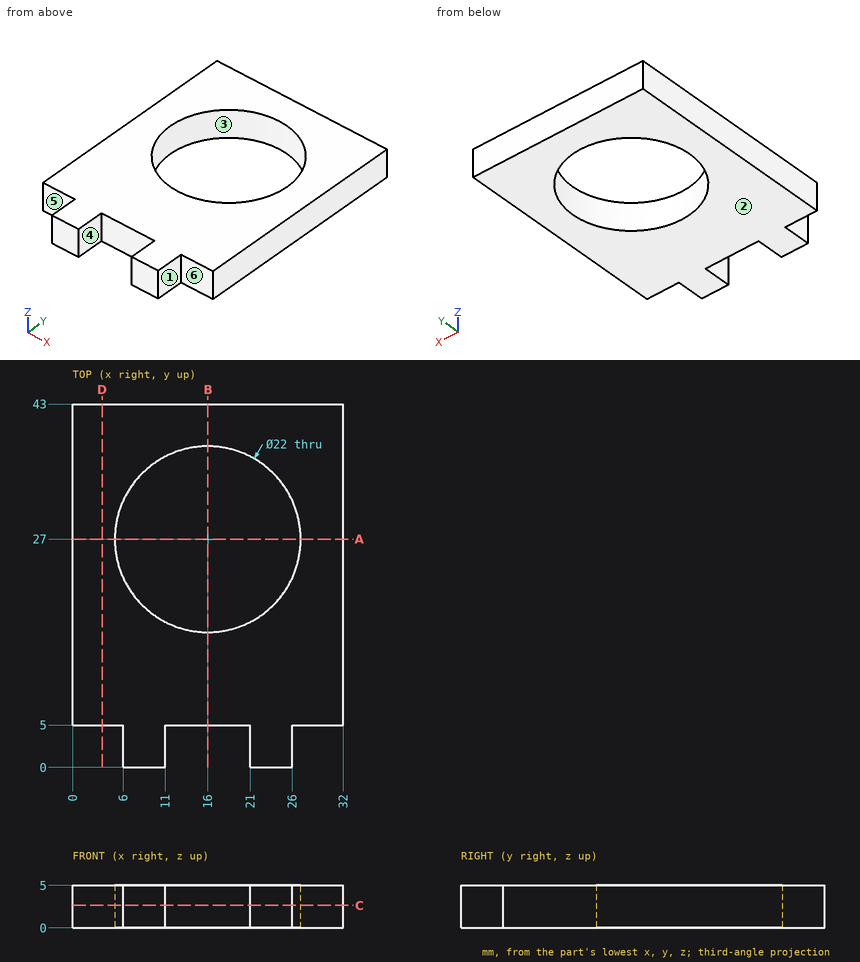
Could you check a few things on this drawing? It's one solid part, dimensions in mm from its lowest x, y, z. A direction names the side the tool comes from. Round coordinates to 2 decimals unless told otherwise and drop trailing zeros. Order: outer loops, then holes, each group sorted by start corner. A loop starts at its lowest first (then second) coordinate and runs counter-clockwise, first axis right, second up. Notation, with made-up numbers: M 19.25,54 L 56.25,54 A18 ccw 56.25,80 Z; hole C 9.5,40.5 d8. An arc over 180 degrees is marked long. One line per question, with ' | ' between items.
1) On a 3-axis mill with a long thin cutter (end or side, diameter ignored), from which of +Z, -Z, +X, -X, +Y, -Y can I reach the whole of each face in a straight line? I mean the marked faces 4, 5 and 6. Say none if no direction works.
Checked values:
face 4: +Z, -Z, -Y | face 5: +Z, -Z, -X, -Y | face 6: +Z, -Z, +X, -Y
2) Imagine slicing it at B-B, the plane x = 16. Write out the boundary of the cut face in (y, z), plus the area to 3 significant figures.
Checked values:
outline: M 5,0 L 16,0 L 16,5 L 5,5 Z; M 38,0 L 43,0 L 43,5 L 38,5 Z | area: 80.0 mm²
3) I need wall thicknesses on line 1 (Y direction, x = 16, z = 2.6); line 2 (X direction, y = 30.5, z = 0.9); line 3 (Y direction, x = 18, z = 4.25). Which ranges of each line are inside material? Lowest first, please.
Checked values:
line 1: y = 5 to 16, 38 to 43 | line 2: x = 0 to 5.57, 26.43 to 32 | line 3: y = 5 to 16.18, 37.82 to 43
4) I'm going to push flat-ended pins straight in: pin 1 Ø2.5 at (y, z) = (2.5, 2) entering from +X; pin 2 Ø2.5 at (y, z) = (3.5, 3) entering from -X. Where does each tip first touch, or does it pass through?
Checked values:
pin 1: stops at x = 26 | pin 2: stops at x = 6
5) We'd pull the mould along X, two halves only. Please class the marked faces 1, 2 and 3: released by +X, released by -X, zero draft, split by the parting line, or undercut.
Checked values:
face 1: released by +X | face 2: zero draft | face 3: undercut
6) Imagine slicing it at C-C, the plane z = 2.65. Write out the boundary of the cut face in (x, y), plus the area to 3 significant figures.
Checked values:
outline: M 0,5 L 6,5 L 6,0 L 11,0 L 11,5 L 21,5 L 21,0 L 26,0 L 26,5 L 32,5 L 32,43 L 0,43 Z; hole C 16,27 d22 | area: 886 mm²
7) Imagine slicing it at D-D, the plane x = 3.5. Write out the boundary of the cut face in (y, z), plus the area to 3 significant figures.
Checked values:
outline: M 5,0 L 43,0 L 43,5 L 5,5 Z | area: 190 mm²
8) Imagine slicing it at A-A, the plane y = 27. Write out the boundary of the cut face in (x, z).
Checked values:
outline: M 0,0 L 5,0 L 5,5 L 0,5 Z; M 27,0 L 32,0 L 32,5 L 27,5 Z
